Design review of the part built by this model. Coordinates are the model's own, in mm. A direction names the side the tool comes from. Coordinates: 2 decimals unless noted, no trailing zeros. Order: outer loops, then holes, each group sorted by start corner. A loop starts at its lowest first (then second) coordinate and runs counter-clockwise, first axis right, second up. Notation, with made-up numbers: (23.5, 70.5) -> (45.5, 70.5) arc R15 cw to (45.5, 85.5) -> close; hole circle Ø1 at (-18, 52). An arc over 180 degrees is marked (long way). Use a Markdown table: item, result. Add a question column.
Q1. Add section C-C (y = 18.5). State the section outline as (x, z) points, then the cut area to 3 significant figures.
Q2. The part is to be moulded in two halves that separate along Y. For faces 3 (the face through (-24, 40, -21)), 4 (the face through (21, -45, -21)), 5 (the face through (-29.97, 0.56, 1.32)), 6 (the face through (23.846, 0.63, 7.509)), say which applies: pulls with the +Y half, pulls with the -Y half, needs draft (parallel to the pull), parting line crosses it, or undercut.
Q3. Add section D-D (z = 87.5). State the section outline as (x, y) points, then the cut area to 3 significant figures.
Q4. Add section A-A (z = 0). State the section outline as (x, y) points, then the cut area to 3 significant figures.
Q5. Wall thickness on probe 1 along Y at (x, z) = (-54.5, 72); probe 2 along Z at (x, y) = (0, 3); probe 3 along X at (y, z) = (-5, 17): over which ranges is each line inside the solid? List them lowest first.
Q6. Machinability: for faces 1 (the face through (95.38, -42.54, 30.04)), 2 (the face through (-24, -40, -21)), which of the approach directions +Z, -Z, +X, -X, +Y, -Y give a long, thin tool a straight path to every point of the face, cutting with its end or side? Answer none if there is none.
Q7. Add section B-B (x = 0). State the section outline as (y, z) points.
Q8. Insertion check: pin 1 (2 mm diameter, centred on y = 4.5, z = 10, fed in from -X); pin 2 (1.5 mm diameter, centred on x = 28.5, y = -13.5, fed in from +Z); pin 3 (1.5 mm diameter, centred on x = -2.5, y = -13, fed in from +Z). Each pin has a flat end and moves straight along its axis. Give the tip position at first contact, or say it passes through.
from build123d import *

# Parameters (mm, degrees)
F0_R     = 100
F0_R_2   = 25
F1_DEPTH = 45
F2_T     = -5


with BuildPart() as f1:
    # F0 (on Front) → F1 (new body, symmetric)
    with BuildSketch(Plane.XZ):
        Circle(F0_R)
        Circle(F0_R_2, mode=Mode.SUBTRACT)
    extrude(amount=F1_DEPTH, both=True)

    # F2
    f2_openings = [f1.faces().sort_by_distance(p)[0] for p in [
        (-100, 0, 0),
    ]]
    offset(amount=F2_T, openings=f2_openings)


solid = f1.part
Established:
| question | item | result |
|---|---|---|
| 1 | outline | circle Ø60 at (0, 0); hole circle Ø50 at (0, 0) |
| 1 | area | 864 mm^2 |
| 2 | face 3 | undercut |
| 2 | face 4 | pulls with the -Y half |
| 2 | face 5 | undercut |
| 2 | face 6 | needs draft |
| 3 | outline | (-48.41, -45) -> (48.41, -45) -> (48.41, -40) -> (-48.41, -40) -> close; (-48.41, 40) -> (48.41, 40) -> (48.41, 45) -> (-48.41, 45) -> close |
| 3 | area | 968 mm^2 |
| 4 | outline | (-100, -45) -> (-25, -45) -> (-25, 45) -> (-100, 45) -> (-100, 40) -> (-30, 40) -> (-30, -40) -> (-100, -40) -> close; (25, -45) -> (100, -45) -> (100, -40) -> (30, -40) -> (30, 40) -> (100, 40) -> (100, 45) -> (25, 45) -> close |
| 4 | area | 2,300 mm^2 |
| 5 | probe 1 | -45 to -40, 40 to 45 |
| 5 | probe 2 | -30 to -25, 25 to 30 |
| 5 | probe 3 | -24.72 to -18.33, 18.33 to 24.72 |
| 6 | face 1 | +Y, -Y |
| 6 | face 2 | none |
| 7 | outline | (-45, -100) -> (-40, -100) -> (-40, -30) -> (40, -30) -> (40, -100) -> (45, -100) -> (45, -25) -> (-45, -25) -> close; (-45, 25) -> (45, 25) -> (45, 100) -> (40, 100) -> (40, 30) -> (-40, 30) -> (-40, 100) -> (-45, 100) -> close |
| 8 | pin 1 | x = -28.62 |
| 8 | pin 2 | z = 11.4 |
| 8 | pin 3 | z = 29.95 |
